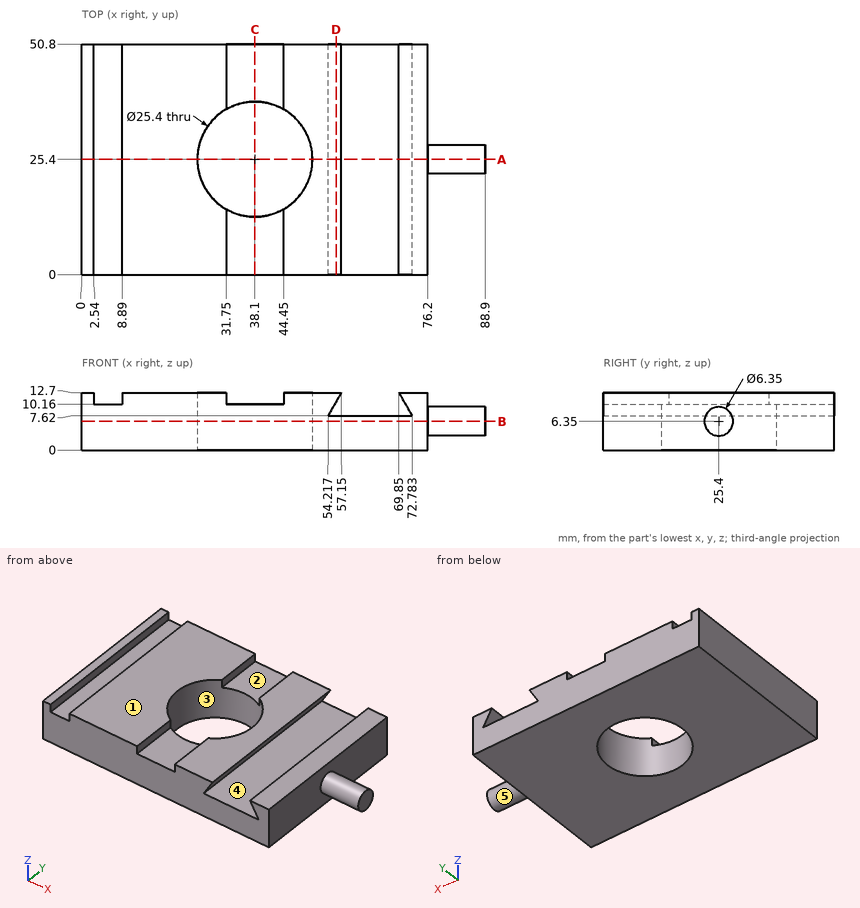
For this review, use the dimensioned drawing (mm, ordinates from the lowest corner) and the shaded views. A direction names the side the tool comes from. Give positions to 0.01 mm unless a question says otherwise; leave off trailing zeros. Order: outer loops, then holes, each group sorted by start corner. A loop starts at its lowest first (then second) coordinate and runs counter-clockwise, first axis right, second up. Notation, with made-up numbers: M 43,-7.75 L 96,-7.75 A31 ccw 96,22.25 Z; hole C 30.25,48.5 d9. An arc over 180 degrees is marked long. One line per question, with ' | ' between items. Start each with the question number.
1) Clearance check with flat-ended pins moving along their axes: P1, Ø3, axis at y = 44, z = 11, coming from the +X side; P2, Ø4, axis at x = 65, y = 40, coming from the +Z side; P3, Ø4, axis at x = 35, y = 46, coming from the +Z side. State where each tip first meets the part, or that it passes through.
2) Consider section A-A, the plane y = 25.4. Give the boundary of the cut face in (x, z) (3 decimals).
3) Wall thickness on L1, parallel to X at y = 25.4, z = 6.25; L2, parallel to X at y = 43.5, z = 11.25; L3, parallel to Y at x = 38.1, z = 2.5: over which ranges is each line inside the solid? List them lowest first. Write a range as from..to.
4) For the marked faces 1 and 2, list the 3-axis set-ups (+Z, -Z, +X, -X, +Y, -Y) from which the entire face can be reached by the end or side of a thin tool; tool diameter is ignored.
5) Consider section D-D, the plane x = 56. Give the boundary of the cut face in (y, z).
6) Consider section B-B, the plane z = 6.35. Give the boundary of the cut face in (x, y) (3 decimals).
7) Consider section C-C, the plane x = 38.1. Give the boundary of the cut face in (y, z).
8) Mouldability with a two-part tool opening along Z and no side actions: class the marked faces 3, 4 and 5 as pulls with the +Z half, pulls with the -Z half, needs draft (parallel to the pull), parting line crosses it, or undercut.
Found:
1) P1: stops at x = 76.2 | P2: stops at z = 7.62 | P3: stops at z = 10.16
2) outline: M 0,0 L 25.4,0 L 25.4,12.7 L 8.89,12.7 L 8.89,10.16 L 2.54,10.16 L 2.54,12.7 L 0,12.7 Z; M 50.8,0 L 76.2,0 L 76.2,3.175 L 88.9,3.175 L 88.9,9.525 L 76.2,9.525 L 76.2,12.7 L 69.85,12.7 L 72.783,7.62 L 54.217,7.62 L 57.15,12.7 L 50.8,12.7 Z
3) L1: x = 0..25.4, 50.8..88.9 | L2: x = 0..2.54, 8.89..31.75, 44.45..56.31, 70.69..76.2 | L3: y = 0..12.7, 38.1..50.8
4) face 1: +Z, +X, -X, +Y, -Y | face 2: +Z, +Y, -Y
5) outline: M 0,0 L 50.8,0 L 50.8,7.62 L 0,7.62 Z; M 0,10.71 L 50.8,10.71 L 50.8,12.7 L 0,12.7 Z
6) outline: M 0,0 L 76.2,0 L 76.2,22.225 L 88.9,22.225 L 88.9,28.575 L 76.2,28.575 L 76.2,50.8 L 0,50.8 Z; hole C 38.1,25.4 d25.4
7) outline: M 0,0 L 12.7,0 L 12.7,10.16 L 0,10.16 Z; M 38.1,0 L 50.8,0 L 50.8,10.16 L 38.1,10.16 Z
8) face 3: needs draft | face 4: undercut | face 5: parting line crosses it
